Model file for the job. Use its own axes, mm. A direction names the side the tool comes from. Round coordinates to 2 decimals unless told otherwise and drop trailing zeros. Loops run counter-clockwise (first coordinate to the right, second up) from the corner with the lowest first, then second, coordinate; pieces in that order, holes last. Notation, with made-up numbers: M 83.5,20 L 140.5,20 A14 cw 140.5,40 Z; hole C -15.5,7.5 d6. An arc over 180 degrees is marked long. Use a Markdown table: item, result. Add a question column.
Q1. Cut at D-D (y = 9.25). Give the cut face in (x, z).
Q2. Tool access for faces 4 (the face through (0.5, 17, 2.5)), 5 (the face through (-2, 17, 0)), 6 (the face through (0, 5, 0)): list every direction of +Z, -Z, +X, -X, +Y, -Y with a clear straight run to the whole face (end or side of a thin tool).
Q3. Mould opens along Z. For faces 1 (the face through (-2.662, 12.082, 1.384)), 2 (the face through (2, 17, 0)), 3 (the face through (1, 10, 0)) say: +Z half, -Z half, draft (parallel to the pull), parting line (faces both ways), or undercut.
Q4. Probe line 1 (Y direction, x = 2, z = -1.7); line 2 (Y direction, x = 0.6, z = 1.8); line 3 (Z direction, x = -0.85, y = 15.5). List the from-to ranges inside material, lowest first. Write a range as from..to.
Q5. Pin check, flat tips, straight feed: pin 1 (1.5 mm diameter, centred on x = 1, z = -2.5, fed in from -Y); pin 2 (0.8 mm diameter, centred on y = 18.5, z = -2.5, fed in from -X); pin 3 (0.8 mm diameter, centred on y = 18, z = -2.5, fed in from +X); pin 4 (1 mm diameter, centred on x = -2, z = -1, fed in from -Y). Stop position of each tip, or through.
Q6. Cut at C-C (x = -1). Give the cut face in (y, z), plus the area to 3 significant figures.
Q7. Cut at A-A (y = 18.5). Give the cut face in (x, z), plus the area to 3 significant figures.
Q8. Cut at B-B (z = 0). Give the cut face in (x, y), plus the area to 3 significant figures.
from build123d import *

# Parameters (mm, degrees)
SKETCH1_R           = 3
BOSS_EXTRUDE1_DEPTH = 20
CUT_EXTRUDE1_DEPTH  = 10
CUT_EXTRUDE2_DEPTH  = 6


with BuildPart() as part:
    # Sketch1 → Boss-Extrude1 (new body)
    with BuildSketch(Plane(origin=(0, 0, 0), x_dir=(1, 0, 0), z_dir=(0, 1, 0))):
        with Locations(Location((0, 0, 0), (0, 0, 270))):
            Circle(SKETCH1_R)
    extrude(amount=BOSS_EXTRUDE1_DEPTH)

    # Sketch2 → Cut-Extrude1 (cut)
    with BuildSketch(Plane.XZ):
        with BuildLine():
            Line((0, 3), (0, -3))
            ThreePointArc((0, -3), (3, 0), (0, 3))
        make_face()
    extrude(amount=-CUT_EXTRUDE1_DEPTH, mode=Mode.SUBTRACT)

    # Sketch3 → Cut-Extrude2 (cut)
    with BuildSketch(Plane(origin=(0, 20, 0), x_dir=(1, 0, 0), z_dir=(0, 1, 0))):
        with BuildLine():
            Line((-0.5, -1.936491673), (-0.5, -3.922731478))
            Line((-0.5, -3.922731478), (0.5, -3.922731478))
            Line((0.5, -3.922731478), (0.5, -1.936491673))
            ThreePointArc((0.5, -1.936491673), (2, 0), (0.5, 1.936491673))
            Line((0.5, 1.936491673), (0.5, 3.922731478))
            Line((0.5, 3.922731478), (-0.5, 3.922731478))
            Line((-0.5, 3.922731478), (-0.5, 1.936491673))
            ThreePointArc((-0.5, 1.936491673), (-2, 0), (-0.5, -1.936491673))
        make_face()
    extrude(amount=-CUT_EXTRUDE2_DEPTH, mode=Mode.SUBTRACT)


solid = part.part
Checked values:
| question | item | result |
|---|---|---|
| 1 | outline | M 0,-3 L 0,3 A3 ccw Z |
| 2 | face 4 | +Z, -Z, +Y |
| 2 | face 5 | +Y |
| 2 | face 6 | +Z, -Z, +X, -Y |
| 3 | face 1 | parting line |
| 3 | face 2 | undercut |
| 3 | face 3 | draft |
| 4 | line 1 | y = 10..20 |
| 4 | line 2 | y = 10..14 |
| 4 | line 3 | z = -2.88..-1.81, 1.81..2.88 |
| 5 | pin 1 | stops at y = 10 |
| 5 | pin 2 | stops at x = -2.14 |
| 5 | pin 3 | stops at x = 2.14 |
| 5 | pin 4 | stops at y = 0 |
| 6 | outline | M 0,-2.83 L 20,-2.83 L 20,-1.73 L 14,-1.73 L 14,1.73 L 20,1.73 L 20,2.83 L 0,2.83 Z |
| 6 | area | 92.4 mm^2 |
| 7 | outline | M -0.5,-2.96 L -0.5,-1.94 A2 cw -0.5,1.94 L -0.5,2.96 A3 ccw Z; M 0.5,-2.96 A3 ccw 0.5,2.96 L 0.5,1.94 A2 cw 0.5,-1.94 Z |
| 7 | area | 13.7 mm^2 |
| 8 | outline | M -3,0 L 0,0 L 0,10 L 3,10 L 3,20 L 2,20 L 2,14 L -2,14 L -2,20 L -3,20 Z |
| 8 | area | 66.0 mm^2 |
